Design review of the part built by this model. Coordinates are the model's own, in mm. A direction names the side the tool comes from. Round coordinates to 2 decimals unless told otherwise and drop trailing zeros. Write each loop counter-clockwise with the first axis right and the second up, starting at its lowest first coordinate (ties: lowest second). Pieces come first, ordered by that corner, then holes.
from build123d import *

# Parameters (mm, degrees)
F0_W     = 890
F0_H     = 420
F1_DEPTH = 25
F3_DEPTH = 25


with BuildPart() as f1:
    # F0 (on Front) → F1 (new body)
    with BuildSketch(Plane.XZ):
        Rectangle(F0_W, F0_H)
    extrude(amount=F1_DEPTH)

    # F2 (on face) → F3 (cut)
    with BuildSketch(Plane.XZ.offset(25)):
        Polygon((-436.426692, -203.834898), (-381.426692, -203.834898), (-326.426692, -203.834898), (-352.426692, 205.339882), (-381.426692, 205.339882), (-410.426692, 205.339882), align=None)
        Polygon((-308.426692, -203.834898), (-253.426692, -203.834898), (-198.426692, -203.834898), (-224.426692, 205.339882), (-253.426692, 205.339882), (-282.426692, 205.339882), align=None)
        Polygon((-180.426692, -203.834898), (-125.426692, -203.834898), (-70.426692, -203.834898), (-96.426692, 205.339882), (-125.426692, 205.339882), (-154.426692, 205.339882), align=None)
        Polygon((-52.426692, -203.834898), (2.573308, -203.834898), (57.573308, -203.834898), (31.573308, 205.339882), (2.573308, 205.339882), (-26.426692, 205.339882), align=None)
        Polygon((75.573308, -203.834898), (130.573308, -203.834898), (185.573308, -203.834898), (159.573308, 205.339882), (130.573308, 205.339882), (101.573308, 205.339882), align=None)
        Polygon((203.573308, -203.834898), (258.573308, -203.834898), (313.573308, -203.834898), (287.573308, 205.339882), (258.573308, 205.339882), (229.573308, 205.339882), align=None)
        Polygon((331.573308, -203.834898), (386.573308, -203.834898), (441.573308, -203.834898), (415.573308, 205.339882), (386.573308, 205.339882), (357.573308, 205.339882), align=None)
    extrude(amount=-F3_DEPTH, mode=Mode.SUBTRACT)


solid = f1.part
1) Add section A-A on x = -116. State the section outline as (y, z) points.
2) The part is to be moulded in two halves that separate along Z. For faces 3 (the face through (-6, -12, 210)), 4 (the face through (259, -13, 205.34)), 5 (the face through (-6, -12, -210)), say which applies: pulls with the +Z half, pulls with the -Z half, needs draft (parallel to the pull), parting line crosses it, or undercut.
3) Add section B-B on y = -7. Count the separate pieces of the cut face and the enclosed holes in it, and give its area (3 significant figures).
4) For line 1 along Z through (x, y) = (361, -17.75), list the stretches that pass through material, from the lowest coordinate up.
5) For faces 1 (the face through (-35, 0, 79)), 2 (the face through (386, -13, -203.835)), list the 3-axis set-ups (+Z, -Z, +X, -X, +Y, -Y) from which the entire face can be reached by the end or side of a thin tool; tool diameter is ignored.
6) Add section D-D on x = 40.5. State the section outline as (y, z) points, and give its area (3 significant figures).
Computed:
1. outline: (-25, -210) - (0, -210) - (0, -203.83) - (-25, -203.83) - close; (-25, 205.34) - (0, 205.34) - (0, 210) - (-25, 210) - close
2. face 3: pulls with the +Z half
2. face 4: undercut
2. face 5: pulls with the -Z half
3. separate pieces: 1
3. enclosed holes: 7
3. area: 133,000 mm2
4. line 1: z = -210 to -203.83, 205.34 to 210
5. face 1: +Z, -Z, +X, -X, +Y
5. face 2: +Y, -Y
6. outline: (-25, -210) - (0, -210) - (0, -203.83) - (-25, -203.83) - close; (-25, 64.86) - (0, 64.86) - (0, 210) - (-25, 210) - close
6. area: 3,780 mm2
